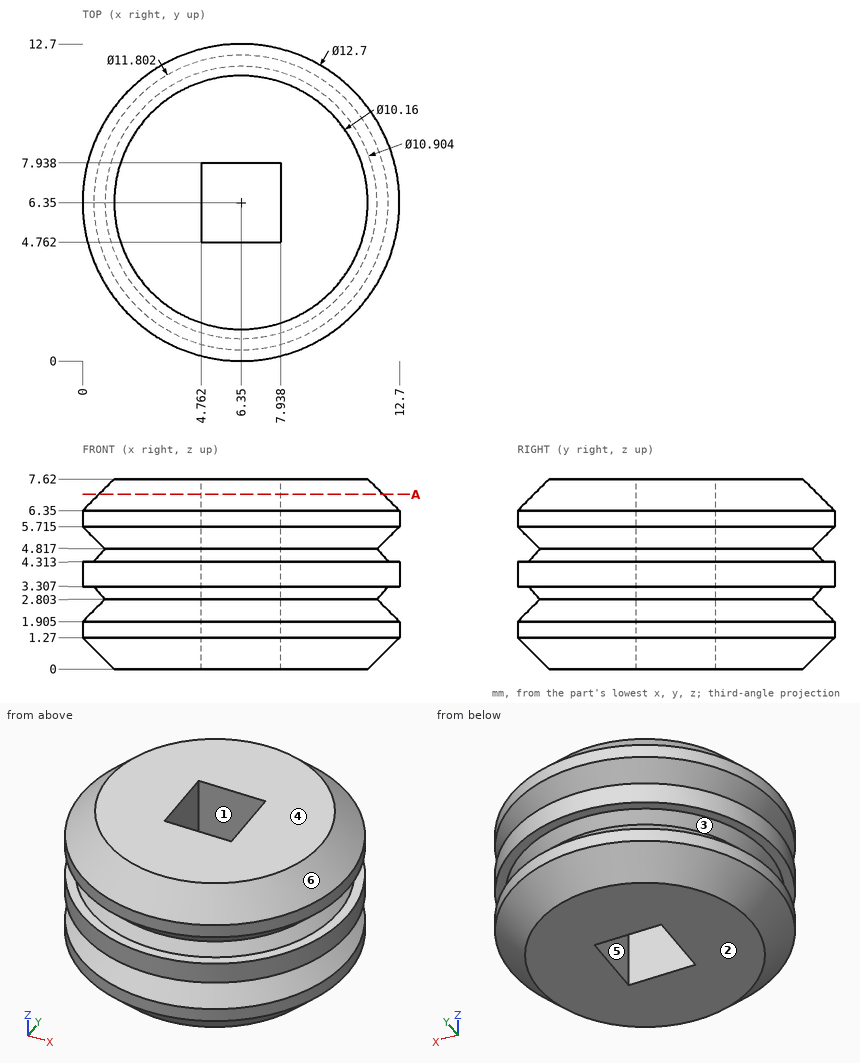
Verification items for this drawing (mm, ordinates from the low corner). A direction names the side the tool comes from. Round coordinates to 2 decimals unless told otherwise and drop trailing zeros. Write each loop counter-clockwise with the first axis right and the second up, starting at its lowest first coordinate (ties: lowest second). Pieces come first, ordered by that corner, then holes. Notation, with made-up numbers: (38, 82) - (62, 82) arc R21 cw to (62, 96) - close; hole circle Ø11 at (-7, 20). An arc over 180 degrees is marked (long way). One line per item, written item: value.
1. Cross-section at A-A on z = 7. Record the boundary of the cut face in (x, y).
The answers:
outline: circle Ø11.4 at (6.35, 6.35); hole (4.76, 4.76) - (7.94, 4.76) - (7.94, 7.94) - (4.76, 7.94) - close
2. Set-up check for the marked faces 1, 2 and 3: record each of +Z, -Z, +X, -X, +Y, -Y from which the full face is reachable in a straight line by a thin tool's end or side.
The answers:
face 1: +Z, -Z
face 2: -Z, +X, -X, +Y, -Y
face 3: none
3. Depth check by flat-ended pin: pin 1 Ø1.5 at (x, z) = (1.5, 2) entering from +Y (1 decimal); pin 2 Ø2 at (x, y) = (5.5, 6.5) entering from -Z; pin 3 Ø1.6 at (x, z) = (7, 5) entering from -Y (1 decimal). Enter the tip coordinate at first touch or a pass-through.
The answers:
pin 1: stops at y = 11.2
pin 2: stops at z = 0
pin 3: stops at y = 0
4. Mould release check, pull along X, two halves, no side actions. Record for the marked faces 4, 5 and 6: released by +X, released by -X, zero draft, split by the parting line, or undercut.
The answers:
face 4: zero draft
face 5: undercut
face 6: split by the parting line
5. Scan lines: L1, parallel to Z at x = 11.25, y = 3 (1 decimal); L2, parallel to Z at x = 2.5, y = 11 (1 decimal); L3, parallel to Y at x = 6.5, z = 6.25. Record each from-to range of solid material in increasing order.
The answers:
L1: z = 0.9 to 2.3, 3.3 to 4.3, 5.3 to 6.8
L2: z = 1 to 2.2, 3.3 to 4.3, 5.4 to 6.7
L3: y = 0 to 4.76, 7.94 to 12.7
